Geometry: final body of the model. Coordinates: model frame, mm. Face numbers are marked on the shaded views. Give positions to 0.01 mm unless a question says otherwise; leave off trailing zeros. Write each loop counter-clockwise with the first axis right and the second up, starting at its lowest first coordinate (ties: lowest second). Pieces come first, ordered by that corner, then holes.
from build123d import *

# Parameters (mm, degrees)
SKETCH1_W           = 228.6
SKETCH1_H           = 69.85
BOSS_EXTRUDE1_DEPTH = 28.702
SKETCH2_R           = 16.002
CUT_EXTRUDE1_DEPTH  = 234.843934843
SKETCH3_R           = 2.286
CUT_EXTRUDE2_DEPTH  = 133.225641813
CUT_EXTRUDE3_DEPTH  = 2.54


with BuildPart() as part:
    # Sketch1 → Boss-Extrude1 (new body)
    with BuildSketch(Plane(origin=(0, 0, 0), x_dir=(1, 0, 0), z_dir=(0, 1, 0))):
        with Locations((8.413464991, -5.090260323)):
            Rectangle(SKETCH1_W, SKETCH1_H)
    extrude(amount=BOSS_EXTRUDE1_DEPTH)

    # Sketch2 → Cut-Extrude1 (cut, through all)
    with BuildSketch(Plane(origin=(122.713464991, 0, 0), x_dir=(0, 0, -1), z_dir=(1, 0, 0))):
        with Locations((-5.090260323, 28.702)):
            Circle(SKETCH2_R)
    extrude(amount=-CUT_EXTRUDE1_DEPTH, mode=Mode.SUBTRACT)

    # Sketch3 → Cut-Extrude2 (cut, through all)
    with BuildSketch(Plane(origin=(0, 28.702, 0), x_dir=(1, 0, 0), z_dir=(0, 1, 0))):
        with Locations(Location((-48.736535009, 18.415261035, 0), (0, 0, 270))):
            Circle(SKETCH3_R)
        with Locations(Location((-48.736535009, -28.595781682, 0), (0, 0, 90))):
            Circle(SKETCH3_R)
        with Locations(Location((65.563464991, 18.415261035, 0), (0, 0, 90))):
            Circle(SKETCH3_R)
        with Locations(Location((65.563464991, -28.595781682, 0), (0, 0, 270))):
            Circle(SKETCH3_R)
    extrude(amount=-CUT_EXTRUDE2_DEPTH, mode=Mode.SUBTRACT)

    # Sketch4 → Cut-Extrude3 (cut)
    with BuildSketch(Plane.XZ):
        Polygon((-49.788475899, 31.090068722), (-47.684271002, 31.090068722), (-46.19637345, 29.602171171), (-46.19637345, 27.497966274), (-47.684271002, 26.010068722), (-49.788475899, 26.010068722), (-51.27637345, 27.497966274), (-51.27637345, 29.602171171), align=None)
        Polygon((-46.19637345, -19.421650524), (-47.684271002, -20.909548076), (-49.788475899, -20.909548076), (-51.27637345, -19.421650524), (-51.27637345, -17.317445628), (-49.788475899, -15.829548076), (-47.684271002, -15.829548076), (-46.19637345, -17.317445628), align=None)
        Polygon((66.615405881, -20.909548076), (64.511200984, -20.909548076), (63.023303432, -19.421650524), (63.023303432, -17.317445628), (64.511200984, -15.829548076), (66.615405881, -15.829548076), (68.103303432, -17.317445628), (68.103303432, -19.421650524), align=None)
        Polygon((63.023303432, 29.602171171), (64.511200984, 31.090068722), (66.615405881, 31.090068722), (68.103303432, 29.602171171), (68.103303432, 27.497966274), (66.615405881, 26.010068722), (64.511200984, 26.010068722), (63.023303432, 27.497966274), align=None)
    extrude(amount=-CUT_EXTRUDE3_DEPTH, mode=Mode.SUBTRACT)


solid = part.part
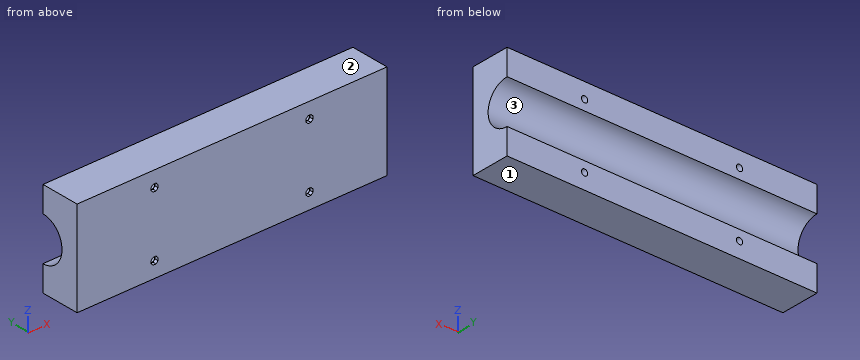
Q1. Section B-B on x = -56. Output: boundary loops of the cut face in (y, z), plus the area to 3 significant figures.
Filled sheet:
outline: (0, -29.83) - (28.7, -29.83) - (28.7, -10.91) arc R16 cw to (28.7, 21.09) - (28.7, 40.02) - (0, 40.02) - close
area: 1,600 mm2
Q2. Pull-direction query (Z, two-part tool) for the marked faces 1, 2 and 3; classes: released by +Z, released by -Z, zero draft, split by the parting line, or undercut.
Filled sheet:
face 1: released by -Z
face 2: released by +Z
face 3: undercut
Q3. Section A-A on y = 20. Output: boundary loops of the cut face in (x, z).
Filled sheet:
outline: (-105.89, -29.83) - (122.71, -29.83) - (122.71, -8.34) - (-105.89, -8.34) - close; (-105.89, 18.52) - (122.71, 18.52) - (122.71, 40.02) - (-105.89, 40.02) - close; hole circle Ø4.57 at (-48.74, -18.42); hole circle Ø4.57 at (-48.74, 28.6); hole circle Ø4.57 at (65.56, -18.42); hole circle Ø4.57 at (65.56, 28.6)
Q4. Section C-C on z = 10. Output: boundary loops of the cut face in (x, y), plus the area to 3 significant figures.
Filled sheet:
outline: (-105.89, 0) - (122.71, 0) - (122.71, 13.47) - (-105.89, 13.47) - close
area: 3,080 mm2
Q5. Pin query (flat end, axial travel): P1, Ø1, axis at y = 25, z = 19.5, coming from the +X side. Return the tip coordinate at first contact, or that it passes through.
Filled sheet:
P1: passes through
Q6. Ray query, line 1 along X through (y, z) = (7, 27.5); line 2 along X through (y, z) = (2, 30); line 3 along Y through (x, z) = (-53, -9). Return the intervals inside material, ascending.
Filled sheet:
line 1: x = -105.89 to -50.74, -46.73 to 63.56, 67.57 to 122.71
line 2: x = -105.89 to -50.88, -46.59 to 63.42, 67.71 to 122.71
line 3: y = 0 to 21.12
